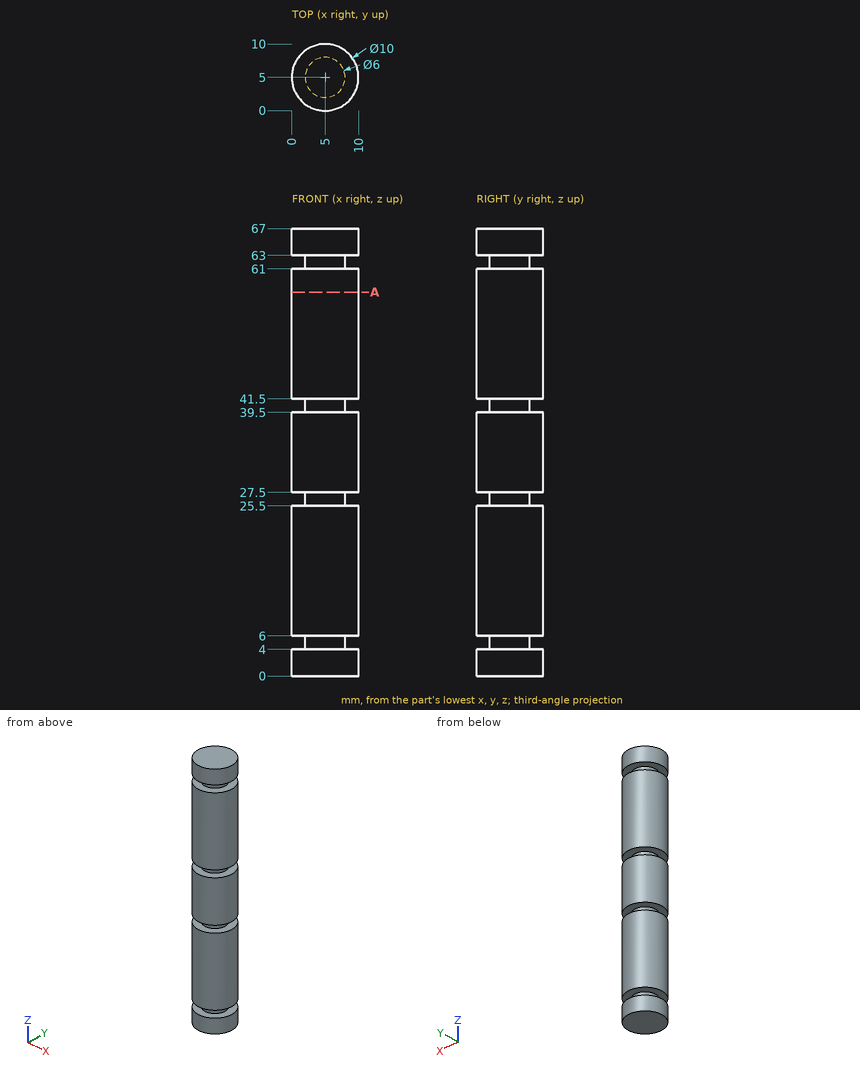
Geometry check sheet. Reference: drawing and pictorial views, mm from the part's lowest x, y, z. Coordinates: 2 decimals unless noted, no trailing zeros. Loops run counter-clockwise (first coordinate to the right, second up) from the corner with the lowest first, then second, coordinate; pieces in that order, holes last. Notation, with made-up numbers: (70, 0) -> (106, 0) arc R37 ccw to (106, 36) -> close; hole circle Ø7 at (30.5, 31). An arc over 180 degrees is marked (long way). Put each result on its own line as item: value.
1) Thickness scan on line 1 (Z direction, x = 2.25, y = 3); line 2 (Y direction, x = 1.5, z = 57.5); line 3 (X direction, y = 2.25, z = 56.5). Record the ranges inside material, lowest first.
Result set:
line 1: z = 0 to 4, 6 to 25.5, 27.5 to 39.5, 41.5 to 61, 63 to 67
line 2: y = 1.43 to 8.57
line 3: x = 0.82 to 9.18
2) Gauge pin test, flat ends, axial feed: pin 1 Ø1.5 at (y, z) = (7.5, 31.5) entering from -X; pin 2 Ø5 at (y, z) = (8, 21.5) entering from -X. Record the tip position at first contact, or that the pin passes through.
Result set:
pin 1: stops at x = 0.32
pin 2: stops at x = 0.03
3) Cross-section at A-A on z = 57.5. Record the boundary of the cut face in (x, y), plus the area to 3 significant figures.
Result set:
outline: circle Ø10 at (5, 5)
area: 78.5 mm^2
